Geometry check sheet. Reference: the model listing, model coordinates, mm. Coordinates: 2 decimals unless noted, no trailing zeros. Write each loop counter-clockwise with the first axis right and the second up, starting at its lowest first coordinate (ties: lowest second). Pieces come first, ordered by that corner, then holes. Notation, with made-up numbers: M 83.25,22 L 133.25,22 A22 ccw 133.25,56 Z; hole C -4.5,73 d10. An arc over 180 degrees is marked long. Put each result on its own line as item: value. Start each with the question number.
1) Scan lines: line 1 along Y through (x, z) = (43, 0.45); line 2 along Y through (x, z) = (59.5, 0.55); line 3 along X through (y, z) = (-11.5, 0.2). Record each from-to range of solid material in increasing order.
2) Cross-section at C-C on z = 0.2. Count the separate pieces of the cut face and the enclosed holes in it, plus the area to 3 significant figures.
3) Cross-section at A-A on x = 37. Record the cut outline in (y, z) (3 decimals).
4) Gauge pin test, flat end, axial feed: pin 1 (4 mm diameter, centred on x = 90, y = -10, fed in from +Z). Record the tip position at first contact, or that the pin passes through.
5) Cross-section at D-D on x = 91. Record the cut outline in (y, z) (3 decimals), plus the area to 3 significant figures.
6) Cross-section at B-B on y = -10. Record the cut outline in (x, z) (3 decimals).
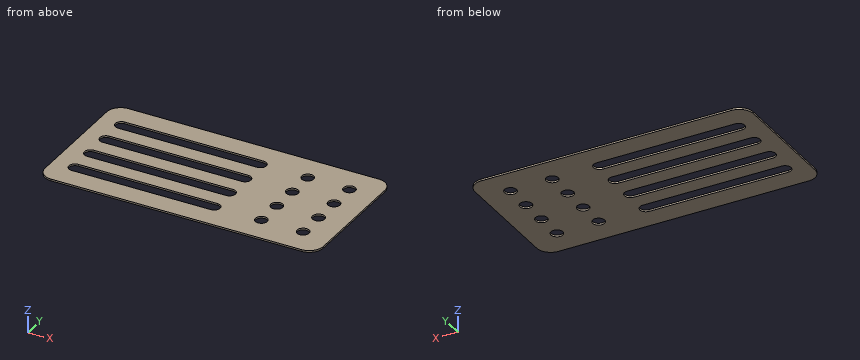
from build123d import *

# Parameters (mm, degrees)
SKETCH1_W           = 100
SKETCH1_H           = 50
SKETCH1_R           = 2.16
BOSS_EXTRUDE1_DEPTH = 0.635
FILLET1_R           = 5


with BuildPart() as part:
    # Sketch1 → Boss-Extrude1 (new body)
    with BuildSketch(Plane.XY):
        with Locations((50, -25)):
            Rectangle(SKETCH1_W, SKETCH1_H)
        with Locations((75, -10)):
            Circle(SKETCH1_R, mode=Mode.SUBTRACT)
        with Locations((90, -10)):
            Circle(SKETCH1_R, mode=Mode.SUBTRACT)
        with Locations((75, -20)):
            Circle(SKETCH1_R, mode=Mode.SUBTRACT)
        with Locations((90, -20)):
            Circle(SKETCH1_R, mode=Mode.SUBTRACT)
        with Locations((75, -30)):
            Circle(SKETCH1_R, mode=Mode.SUBTRACT)
        with Locations((90, -30)):
            Circle(SKETCH1_R, mode=Mode.SUBTRACT)
        with Locations((75, -40)):
            Circle(SKETCH1_R, mode=Mode.SUBTRACT)
        with Locations((90, -40)):
            Circle(SKETCH1_R, mode=Mode.SUBTRACT)
        with BuildLine():
            Line((8, -7.84), (58, -7.84))
            ThreePointArc((58, -7.84), (60.16, -10), (58, -12.16))
            Line((58, -12.16), (8, -12.16))
            ThreePointArc((8, -12.16), (5.84, -10), (8, -7.84))
        make_face(mode=Mode.SUBTRACT)
        with BuildLine():
            Line((8, -22.16), (58, -22.16))
            ThreePointArc((58, -22.16), (60.16, -20), (58, -17.84))
            Line((58, -17.84), (8, -17.84))
            ThreePointArc((8, -17.84), (5.84, -20), (8, -22.16))
        make_face(mode=Mode.SUBTRACT)
        with BuildLine():
            Line((8, -32.16), (58, -32.16))
            ThreePointArc((58, -32.16), (60.16, -30), (58, -27.84))
            Line((58, -27.84), (8, -27.84))
            ThreePointArc((8, -27.84), (5.84, -30), (8, -32.16))
        make_face(mode=Mode.SUBTRACT)
        with BuildLine():
            Line((8, -42.16), (58, -42.16))
            ThreePointArc((58, -42.16), (60.16, -40), (58, -37.84))
            Line((58, -37.84), (8, -37.84))
            ThreePointArc((8, -37.84), (5.84, -40), (8, -42.16))
        make_face(mode=Mode.SUBTRACT)
    extrude(amount=BOSS_EXTRUDE1_DEPTH)

    # Fillet1
    fillet1_edges = [part.edges().sort_by_distance(p)[0] for p in [
        (100, 0, 0.3175),
        (100, -50, 0.3175),
        (0, -50, 0.3175),
        (0, 0, 0.3175),
    ]]
    fillet(fillet1_edges, radius=FILLET1_R)


solid = part.part
Answer key:
1. line 1: y = -50 to -42.16, -37.84 to -32.16, -27.84 to -22.16, -17.84 to -12.16, -7.84 to 0
1. line 2: y = -50 to -41.55, -38.45 to -31.55, -28.45 to -21.55, -18.45 to -11.55, -8.45 to 0
1. line 3: x = 0 to 6.45, 59.55 to 73.45, 76.55 to 88.45, 91.55 to 100
2. separate pieces: 1
2. enclosed holes: 12
2. area: 3,940 mm²
3. outline: M -50,0 L -42.16,0 L -42.16,0.635 L -50,0.635 Z; M -37.84,0 L -32.16,0 L -32.16,0.635 L -37.84,0.635 Z; M -27.84,0 L -22.16,0 L -22.16,0.635 L -27.84,0.635 Z; M -17.84,0 L -12.16,0 L -12.16,0.635 L -17.84,0.635 Z; M -7.84,0 L 0,0 L 0,0.635 L -7.84,0.635 Z
4. pin 1: passes through
5. outline: M -50,0 L -41.915,0 L -41.915,0.635 L -50,0.635 Z; M -38.085,0 L -31.915,0 L -31.915,0.635 L -38.085,0.635 Z; M -28.085,0 L -21.915,0 L -21.915,0.635 L -28.085,0.635 Z; M -18.085,0 L -11.915,0 L -11.915,0.635 L -18.085,0.635 Z; M -8.085,0 L 0,0 L 0,0.635 L -8.085,0.635 Z
5. area: 22.0 mm²
6. outline: M 0,0 L 5.84,0 L 5.84,0.635 L 0,0.635 Z; M 60.16,0 L 72.84,0 L 72.84,0.635 L 60.16,0.635 Z; M 77.16,0 L 87.84,0 L 87.84,0.635 L 77.16,0.635 Z; M 92.16,0 L 100,0 L 100,0.635 L 92.16,0.635 Z
